from build123d import *

# Parameters (mm, degrees)
F1_DEPTH  = 25.4
F2_R      = 5.08
F4_DEPTH  = 10.16
F6_DEPTH  = 10.16
F7_R      = 6.35
F8_DEPTH  = 50.8
F10_W     = 76.8076643543
F10_H     = 11.4133090087
F11_DEPTH = 7.62
F13_R     = 8.89
F14_DEPTH = 179.578
F16_R     = 1.27
F17_DEPTH = 60.198


# Not quite as in the source:
# - a feature names something its author has since deleted; it is built from what else it names


with BuildPart() as f1:
    # F0 (on Right) → F1 (new body, symmetric)
    with BuildSketch(Plane.YZ):
        Polygon((-60.8564667081, 20.32), (-76.0964667081, 0), (50.9035332919, 0), (50.9035332919, 20.32), (40.7435332919, 33.02), (-2.4364667081, 33.02), (-27.8364667081, 20.32), align=None)
    extrude(amount=F1_DEPTH, both=True)

    # F2
    f2_edges = [f1.edges().sort_by_distance(p)[0] for p in [
        (25.4, -68.476467, 10.16),
        (25.4, -44.346467, 20.32),
        (25.4, -15.136467, 26.67),
        (25.4, 19.153533, 33.02),
        (25.4, 45.823533, 26.67),
        (25.4, 50.903533, 10.16),
        (0, 50.903533, 20.32),
        (0, 40.743533, 33.02),
        (0, -60.856467, 20.32),
        (0, -27.836467, 20.32),
        (0, -2.436467, 33.02),
        (-25.4, -15.136467, 26.67),
        (-25.4, -44.346467, 20.32),
        (-25.4, -68.476467, 10.16),
        (-25.4, 19.153533, 33.02),
        (-25.4, 50.903533, 10.16),
        (-25.4, 45.823533, 26.67),
    ]]
    fillet(f2_edges, radius=F2_R)

    # F3 (on face) → F4 (cut)
    with BuildSketch(Plane.YZ.offset(25.4)):
        with BuildLine():
            Line((-60.8564667081, 0), (-35.4564667081, 0))
            ThreePointArc((-35.4564667081, 0), (-48.1564667081, 12.7), (-60.8564667081, 0))
        make_face()
        with BuildLine():
            ThreePointArc((40.7435332919, 0), (28.0435332919, 12.7), (15.3435332919, 0))
            Line((15.3435332919, 0), (40.7435332919, 0))
        make_face()
    extrude(amount=-F4_DEPTH, mode=Mode.SUBTRACT)

    # F5 (on face) → F6 (cut)
    with BuildSketch(Plane(origin=(-25.4, 0, 0), x_dir=(0, -1, 0), z_dir=(-1, 0, 0))):
        with BuildLine():
            Line((-40.7435332919, 0), (-15.3435332919, 0))
            ThreePointArc((-15.3435332919, 0), (-28.0435332919, 12.7), (-40.7435332919, 0))
        make_face()
        with BuildLine():
            Line((35.4564667081, 0), (60.8564667081, 0))
            ThreePointArc((60.8564667081, 0), (48.1564667081, 12.7), (35.4564667081, 0))
        make_face()
    extrude(amount=-F6_DEPTH, mode=Mode.SUBTRACT)

    # F7 (on face) → F8 (join)
    with BuildSketch(Plane.YZ.offset(15.24)):
        with BuildLine():
            Line((32.2078052294, 0), (24.5878052294, 0))
            ThreePointArc((24.5878052294, 0), (28.3978052294, -1.27), (32.2078052294, 0))
        make_face()
        with Locations((-48.3666342305, 5.08)):
            Circle(F7_R)
        with BuildLine():
            ThreePointArc((32.2078052294, 0), (34.0774178922, 2.2401936686), (34.7478052294, 5.08))
            ThreePointArc((34.7478052294, 5.08), (25.5579988979, 10.7596126628), (24.5878052294, 0))
            Line((24.5878052294, 0), (32.2078052294, 0))
        make_face()
    extrude(amount=F8_DEPTH)

    # F9: F1 across plane


with BuildPart() as f1_1:
    add(f1.part)
    add(f1.part.mirror(Plane.YZ))

    # F10 (on face) → F11 (join)
    with BuildSketch(Plane.YZ.offset(66.04)):
        with Locations((-9.5459215246, 4.4366544964)):
            Rectangle(F10_W, F10_H)
    extrude(amount=F11_DEPTH)

    # F12: F1 across plane


with BuildPart() as f1_2:
    add(f1_1.part)
    add(f1_1.part.mirror(Plane.YZ))

    # F13 (on face) → F14 (join)
    with BuildSketch(Plane.YZ.offset(73.66)):
        with Locations((-9.5459241474, 3.0935325194)):
            Circle(F13_R)
    extrude(amount=F14_DEPTH)

    # F15: F1 across plane


with BuildPart() as f1_3:
    add(f1_2.part)
    add(f1_2.part.mirror(Plane.YZ))

    # F16 (on face) → F17 (join)
    with BuildSketch(Plane.XY.offset(33.02)):
        with Locations((0, 6.6220072263)):
            Circle(F16_R)
    extrude(amount=F17_DEPTH)


solid = f1_3.part
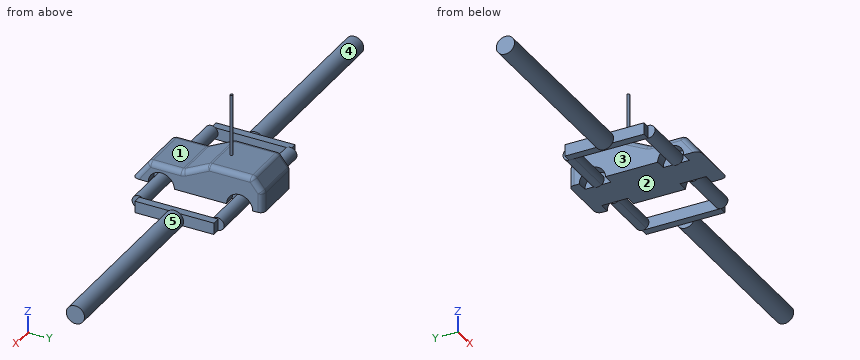
Read the model definition and answer for the solid it produces. Units are mm, in the model's axes. Face numbers are marked on the shaded views. A direction names the side the tool comes from. Give positions to 0.01 mm unless a question says otherwise; leave off trailing zeros. Write each loop counter-clockwise with the first axis right and the second up, starting at its lowest first coordinate (ties: lowest second). Pieces come first, ordered by that corner, then holes. Notation, with made-up numbers: (66.25, 62.5) -> (71.25, 62.5) arc R24 ccw to (71.25, 94.5) -> close; hole circle Ø4 at (1.25, 74.5). An arc over 180 degrees is marked (long way). Answer as a JSON object with one key per item and string values. Group by question number.
1) Each of these flat-tipped pins is pushed along its axis until it touches: P1, Ø1.5, axis at x = -162, y = -13.5, coming from the -Z side; P2, Ø1, axis at y = 11.5, z = 35, coming from the -X side; P3, Ø4, axis at x = -68.5, z = 3.5, coming from the -Y side; P4, Ø3, axis at y = 31, z = 4.5, coming from the +X side. Where does it stop, or does it pass through?
2) Consider L1, parallel to X at y = -14.5, z = 8; L2, parallel to X at y = -49.5, z = 16; L3, parallel to Z at x = 109, y = -10. Determine where each line is inside the solid, lowest interval first. Write a range as from..to.
3) Find section B-B (x = 83). Write down the section's boundary in (y, z), and give its area (3 significant figures).
4) Find section A-A (z = 66). Write down the section's boundary in (x, y), and give its area (3 significant figures).
5) A tool of negligible diameter and unlimited length cuts with its end or side. For the marked faces 3, 4 and 5, from which of +Z, -Z, +X, -X, +Y, -Y can it reach the whole face along a straight path? Write none if from no direction.
6) The mould has two halves that part along X. Classify the marked faces 1 and 2: +X half, -X half, draft (parallel to the pull), parting line (faces both ways), or undercut.
Values follow:
{
 "1": {"P1": "stops at z = -5.2", "P2": "passes through", "P3": "stops at y = -47.95", "P4": "stops at x = 66.04"},
 "2": {"L1": "x = -253.24..-66.04, -25.4..25.4, 66.04..253.24", "L2": "x = -25.34..25.34", "L3": "z = -5.78..11.97"},
 "3": {"outline": "circle Ø17.78 at (-9.55, 3.09)", "area": "248 mm2"},
 "4": {"outline": "circle Ø2.54 at (0, 6.62)", "area": "5.07 mm2"},
 "5": {"face 3": "+Z", "face 4": "-X", "face 5": "+X"},
 "6": {"face 1": "draft", "face 2": "undercut"}
}
